Geometry: see drawing. Coordinates: mm, zero at the bounding-box minimum. A direction names the side the tool comes from. Round coordinates to 2 decimals unless told otherwise and drop trailing zeros. Order: outer loops, then holes, each group sorted by start corner. A loop starts at its lowest first (then second) coordinate and runs counter-clockwise, first axis right, second up. Notation, with made-up numbers: (44.5, 51) -> (77.5, 51) arc R17 ccw to (77.5, 57) -> close; hole circle Ø9 at (-32.75, -5). An arc over 180 degrees is marked (long way). Use a Markdown table: item, result.
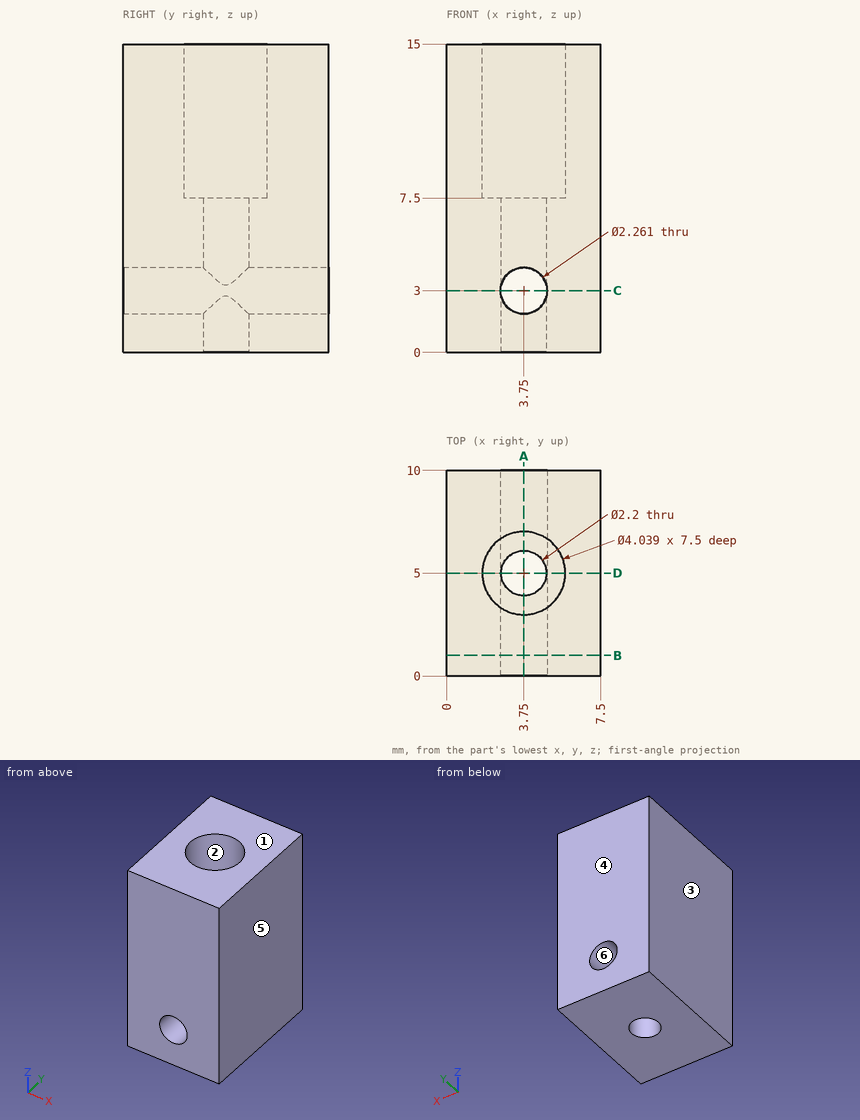
1) Draft query along X for the marked faces 3, 4, 5 and 6. Return one class per face: released by +X, released by -X, zero draft, split by the parting line, or undercut.
Answer key:
| item | result |
|---|---|
| face 3 | released by -X |
| face 4 | zero draft |
| face 5 | released by +X |
| face 6 | undercut |
2) Cut plane A-A on x = 3.75. Return loops of the section in (y, z).
Answer key:
| item | result |
|---|---|
| outline | (0, 0) -> (3.9, 0) -> (3.9, 1.87) -> (0, 1.87) -> close; (0, 4.13) -> (3.9, 4.13) -> (3.9, 7.5) -> (2.98, 7.5) -> (2.98, 15) -> (0, 15) -> close; (6.1, 0) -> (10, 0) -> (10, 1.87) -> (6.1, 1.87) -> close; (6.1, 4.13) -> (10, 4.13) -> (10, 15) -> (7.02, 15) -> (7.02, 7.5) -> (6.1, 7.5) -> close |
3) Ray query, probe 1 along Y at (x, z) = (3.75, 4.95); probe 2 along Y at (x, z) = (3.75, 11.75); probe 3 along Z at (x, y) = (5.25, 3.75). Return the intervals inside material, ascending.
Answer key:
| item | result |
|---|---|
| probe 1 | y = 0 to 3.9, 6.1 to 10 |
| probe 2 | y = 0 to 2.98, 7.02 to 10 |
| probe 3 | z = 0 to 7.5 |
4) Cut plane B-B on y = 1. Return loops of the section in (x, z).
Answer key:
| item | result |
|---|---|
| outline | (0, 0) -> (7.5, 0) -> (7.5, 15) -> (0, 15) -> close; hole circle Ø2.26 at (3.75, 3) |
5) Cut plane D-D on y = 5. Return loops of the section in (x, z).
Answer key:
| item | result |
|---|---|
| outline | (0, 0) -> (2.65, 0) -> (2.65, 2.74) arc R1.13 cw to (2.65, 3.26) -> (2.65, 7.5) -> (1.73, 7.5) -> (1.73, 15) -> (0, 15) -> close; (4.85, 0) -> (7.5, 0) -> (7.5, 15) -> (5.77, 15) -> (5.77, 7.5) -> (4.85, 7.5) -> (4.85, 3.26) arc R1.13 cw to (4.85, 2.74) -> close |
6) Contact query for flat-ended pins moving along their axis: P1, Ø1.2, axis at x = 4, y = 5, coming from the +Z side; P2, Ø2.5, axis at x = 3.75, y = 5, coming from the +Z side. Output: stop coordinate, or through.
Answer key:
| item | result |
|---|---|
| P1 | passes through |
| P2 | stops at z = 7.5 |
7) Cut plane C-C on z = 3. Return loops of the section in (x, y).
Answer key:
| item | result |
|---|---|
| outline | (0, 0) -> (2.62, 0) -> (2.62, 10) -> (0, 10) -> close; (4.88, 0) -> (7.5, 0) -> (7.5, 10) -> (4.88, 10) -> close |
8) Set-up query: the marked faces 1 and 2. Return all of +Z, -Z, +X, -X, +Y, -Y with unobstructed straight access to the full face (end or side cutting, diameter ignored); none if empty.
Answer key:
| item | result |
|---|---|
| face 1 | +Z, +X, -X, +Y, -Y |
| face 2 | +Z |
